```python
from build123d import *

# Parameters (mm, degrees)
F0_R     = 15
F0_R_2   = 10
F1_DEPTH = 25
F2_DEPTH = 50
F3_R     = 5
F4_SIZE  = 3


with BuildPart() as f1:
    # F0 (on Front) → F1 (new body)
    with BuildSketch(Plane.XZ):
        with BuildLine():
            ThreePointArc((6.25, -29.341736), (23.318448, -18.874586), (30, 0))
            ThreePointArc((30, 0), (23.318448, 18.874586), (6.25, 29.341736))
            ThreePointArc((6.25, 29.341736), (-30, 0), (6.25, -29.341736))
        make_face()
        Circle(F0_R, mode=Mode.SUBTRACT)
        with BuildLine():
            ThreePointArc((6.25, 29.341736), (23.318448, 18.874586), (30, 0))
            ThreePointArc((30, 0), (23.318448, -18.874586), (6.25, -29.341736))
            Line((6.25, -29.341736), (63.645833, -17.116013))
            ThreePointArc((63.645833, -17.116013), (42.5, 0), (63.645833, 17.116013))
            Line((63.645833, 17.116013), (6.25, 29.341736))
        make_face()
        with BuildLine():
            ThreePointArc((77.5, 0), (73.602428, 11.010175), (63.645833, 17.116013))
            ThreePointArc((63.645833, 17.116013), (42.5, 0), (63.645833, -17.116013))
            ThreePointArc((63.645833, -17.116013), (73.602428, -11.010175), (77.5, 0))
        make_face()
        with Locations((60, 0)):
            Circle(F0_R_2, mode=Mode.SUBTRACT)
    extrude(amount=F1_DEPTH)

    # F0 (on Front) → F2 (join)
    with BuildSketch(Plane.XZ):
        with BuildLine():
            ThreePointArc((6.25, -29.341736), (23.318448, -18.874586), (30, 0))
            ThreePointArc((30, 0), (23.318448, 18.874586), (6.25, 29.341736))
            ThreePointArc((6.25, 29.341736), (-30, 0), (6.25, -29.341736))
        make_face()
        Circle(F0_R, mode=Mode.SUBTRACT)
    extrude(amount=F2_DEPTH)

    # F3
    f3_edges = [f1.edges().sort_by_distance(p)[0] for p in [
        (-6.25, -50, 29.341736),
    ]]
    fillet(f3_edges, radius=F3_R)

    # F4
    f4_edges = [f1.edges().sort_by_distance(p)[0] for p in [
        (-15, -50, 0),
        (50, -25, 0),
    ]]
    chamfer(f4_edges, length=F4_SIZE)


solid = f1.part
```
The model under review builds one solid part; all positions refer to its coordinate system, in mm. Coordinates: 2 decimals unless noted, no trailing zeros. Write each loop counter-clockwise with the first axis right and the second up, starting at its lowest first coordinate (ties: lowest second). Pieces come first, ordered by that corner, then holes.
1) The part is to be moulded in two halves that separate along X. For faces 1 (the face through (34.546, -12.325, -23.314)), 2 (the face through (49.86, -22.15, 0.45)), 3 (the face through (23, 0, 0)), say which applies: pulls with the +X half, pulls with the -X half, needs draft (parallel to the pull), parting line crosses it, or undercut.
2) We need section A-A on y = -3. State the section outline as (x, z) points, then the cut area to 3 significant figures.
3) To check wall thickness, follow probe 1 along Z at (x, y) = (0, -33); probe 2 along X at (y, z) = (-15, 1.5); probe 3 along Z at (x, y) = (60, -9). State the ranges of each line that lie inside material, in increasing order.
4) Clearance check with flat-ended pins moving along their axes: pin 1 Ø6 at (y, z) = (-28.5, 0) entering from -X; pin 2 Ø2 at (x, y) = (-11.5, -12.5) entering from +Z; pin 3 Ø6 at (x, y) = (47.5, -24) entering from +Z. State where each tip first meets the part, or that it passes through.
5) We need section C-C on y = -43.5. State the section outline as (x, z) points, then the cut area to 3 significant figures.
6) We need section B-B on x = 60. State the section outline as (y, z) points, then the cut area to 3 significant figures.
7) We need section D-D on z = 1.5. Count the separate pieces of the cut face and the enclosed holes in it, then the cut area to 3 significant figures.
Answer list:
1. face 1: pulls with the +X half
1. face 2: undercut
1. face 3: needs draft
2. outline: (6.25, -29.34) - (63.65, -17.12) arc R17.5 ccw to (63.65, 17.12) - (6.25, 29.34) arc R30 ccw (long way) to start; hole circle Ø30 at (0, 0); hole circle Ø20 at (60, 0)
2. area: 3,790 mm2
3. probe 1: z = -30 to -15, 15 to 30
3. probe 2: x = -29.96 to -14.92, 14.92 to 50.11, 69.89 to 77.44
3. probe 3: z = -17.89 to -10, 10 to 17.89
4. pin 1: stops at x = -30
4. pin 2: stops at z = 28.1
4. pin 3: stops at z = 21.19
5. outline: (6.25, -29.34) arc R30 ccw to (30, 0) arc R30 ccw to (6.25, 29.34) arc R30 ccw (long way) to start; hole circle Ø30 at (0, 0)
5. area: 2,120 mm2
6. outline: (-25, -17.89) - (0, -17.89) - (0, -10) - (-22, -10) - (-25, -13) - close; (-25, 13) - (-22, 10) - (0, 10) - (0, 17.89) - (-25, 17.89) - close
6. area: 386 mm2
7. separate pieces: 3
7. enclosed holes: 0
7. area: 2,170 mm2
